Verification items for the finished model (mm, model axes). Coordinates: 2 decimals unless noted, no trailing zeros. Loops run counter-clockwise (first coordinate to the right, second up) from the corner with the lowest first, then second, coordinate; pieces in that order, holes last. Notation, with made-up numbers: (-5.5, 52.25) -> (48.5, 52.25) arc R32 cw to (48.5, 90.25) -> close; hole circle Ø3 at (-10.5, 43.5). An arc over 180 degrees is marked (long way). Answer as a JSON object with one key per item and string values. Group by question number.
Q1. Cross-section at A-A on z = 32.5. Record the boundary of the cut face in (x, y), and give its area (3 significant figures).
Q2. Cross-section at C-C on y = 1.8. Give the number of separate pieces and of enclosed holes in the cut face, and give its area (3 significant figures).
Q3. Scan lines: L1, parallel to X at y = 1.2, z = -29; L2, parallel to X at y = 0.6, z = 9; L3, parallel to X at y = 0.7, z = -32.5. Record each from-to range of solid material in increasing order.
Q4. Gauge pin test, flat ends, axial feed: pin 1 Ø6.5 at (x, z) = (-42.5, 32.5) entering from +Y; pin 2 Ø0.8 at (y, z) = (1, 3) entering from -X; pin 3 Ø1 at (y, z) = (1.5, -0.5) entering from +X; pin 4 Ø0.8 at (x, y) = (2, 1) entering from +Z. Record the tip position at first contact, or that the pin passes through.
Q5. Cross-section at B-B on x = 42.5. Record the boundary of the cut face in (y, z).
```python
from build123d import *

# Parameters (mm, degrees)
EXTRUDE_1_DEPTH     = 2.5
SKETCH_3_R          = 2
CUT_EXTRUDE_1_DEPTH = 61.570207198
CUT_EXTRUDE_2_DEPTH = 61.570207198
FILLET_1_R          = 2
FILLET_2_R          = 2


with BuildPart() as part:
    # 草图2 → 凸台-拉伸1 (new body)
    with BuildSketch(Plane(origin=(0, 0, 0), x_dir=(1, 0, 0), z_dir=(0, 1, 0))):
        Polygon((-47.5, 37.5), (-30.5, 37.5), (-20, 27), (20, 27), (30.5, 37.5), (47.5, 37.5), (47.5, 26.521871089), (36.45, 22.5), (36.45, -22.5), (47.5, -26.521871089), (47.5, -37.5), (30.5, -37.5), (20, -27), (-20, -27), (-30.5, -37.5), (-47.5, -37.5), (-47.5, -26.521871089), (-36.45, -22.5), (-36.45, 22.5), (-47.5, 26.521871089), align=None)
    extrude(amount=EXTRUDE_1_DEPTH)

    # 草图3 → 切除-拉伸1 (cut, through all)
    with BuildSketch(Plane(origin=(0, 2.5, 0), x_dir=(1, 0, 0), z_dir=(0, 1, 0))):
        with Locations(Location((-42.5, -32.5, 0), (0, 0, 270))):
            Circle(SKETCH_3_R)
        with Locations(Location((42.5, -32.5, 0), (0, 0, 270))):
            Circle(SKETCH_3_R)
        with Locations(Location((42.5, 32.5, 0), (0, 0, 90))):
            Circle(SKETCH_3_R)
        with Locations(Location((-42.5, 32.5, 0), (0, 0, 90))):
            Circle(SKETCH_3_R)
    extrude(amount=-CUT_EXTRUDE_1_DEPTH, mode=Mode.SUBTRACT)

    # 草图4 → 切除-拉伸2 (cut, through all)
    with BuildSketch(Plane(origin=(0, 2.5, 0), x_dir=(1, 0, 0), z_dir=(0, 1, 0))):
        with BuildLine():
            Line((14.432710429, 17.261137554), (0, 2.828427125))
            Line((0, 2.828427125), (-14.432710429, 17.261137554))
            ThreePointArc((-14.432710429, 17.261137554), (0, 22.5), (14.432710429, 17.261137554))
        make_face()
        with BuildLine():
            Line((17.261137554, 14.432710429), (2.828427125, 0))
            Line((2.828427125, 0), (17.261137554, -14.432710429))
            ThreePointArc((17.261137554, -14.432710429), (22.5, 0), (17.261137554, 14.432710429))
        make_face()
        with BuildLine():
            Line((14.432710429, -17.261137554), (0, -2.828427125))
            Line((0, -2.828427125), (-14.432710429, -17.261137554))
            ThreePointArc((-14.432710429, -17.261137554), (0, -22.5), (14.432710429, -17.261137554))
        make_face()
        with BuildLine():
            Line((-17.261137554, 14.432710429), (-2.828427125, 0))
            Line((-2.828427125, 0), (-17.261137554, -14.432710429))
            ThreePointArc((-17.261137554, -14.432710429), (-22.5, 0), (-17.261137554, 14.432710429))
        make_face()
        Polygon((-17.261137554, 25.402553145), (-34.014066988, 5.737935313), (-26.260100349, 5.737935313), align=None)
        Polygon((-32.876818547, 14.112219282), (-26.260100349, 27), (-32.876818547, 33.858987655), align=None)
        Polygon((26.260100349, 27), (32.876818547, 33.858987655), (32.876818547, 14.112219282), align=None)
        Polygon((34.014066988, 5.737935313), (26.260100349, 5.737935313), (17.261137554, 25.402553145), align=None)
        Polygon((32.876818547, -14.112219282), (26.260100349, -27), (32.876818547, -33.858987655), align=None)
        Polygon((17.261137554, -25.402553145), (34.014066988, -5.737935313), (26.260100349, -5.737935313), align=None)
        Polygon((-26.260100349, -27), (-32.876818547, -33.858987655), (-32.876818547, -14.112219282), align=None)
        Polygon((-34.014066988, -5.737935313), (-26.260100349, -5.737935313), (-17.261137554, -25.402553145), align=None)
    extrude(amount=-CUT_EXTRUDE_2_DEPTH, mode=Mode.SUBTRACT)

    # 圆角1
    fillet_1_edges = [part.edges().sort_by_distance(p)[0] for p in [
        (-32.876818547, 1.25, -14.112219282),
        (-32.876818547, 1.25, -33.858987655),
        (-26.260100349, 1.25, -27),
        (32.876818547, 1.25, -14.112219282),
        (26.260100349, 1.25, -27),
        (32.876818547, 1.25, -33.858987655),
        (17.261137554, 1.25, -25.402553145),
        (34.014066988, 1.25, -5.737935313),
        (26.260100349, 1.25, -5.737935313),
        (32.876818547, 1.25, 14.112219282),
        (32.876818547, 1.25, 33.858987655),
        (26.260100349, 1.25, 27),
        (14.432710429, 1.25, 17.261137554),
        (-14.432710429, 1.25, 17.261137554),
        (0, 1.25, 2.828427125),
        (17.261137554, 1.25, -14.432710429),
        (17.261137554, 1.25, 14.432710429),
        (2.828427125, 1.25, 0),
        (-17.261137554, 1.25, -25.402553145),
        (-26.260100349, 1.25, -5.737935313),
        (-34.014066988, 1.25, -5.737935313),
        (-17.261137554, 1.25, 14.432710429),
        (-17.261137554, 1.25, -14.432710429),
        (-2.828427125, 1.25, 0),
        (-17.261137554, 1.25, 25.402553145),
        (-34.014066988, 1.25, 5.737935313),
        (-26.260100349, 1.25, 5.737935313),
        (-32.876818547, 1.25, 14.112219282),
        (-26.260100349, 1.25, 27),
        (-32.876818547, 1.25, 33.858987655),
        (17.261137554, 1.25, 25.402553145),
        (26.260100349, 1.25, 5.737935313),
        (34.014066988, 1.25, 5.737935313),
        (-14.432710429, 1.25, -17.261137554),
        (14.432710429, 1.25, -17.261137554),
        (0, 1.25, -2.828427125),
    ]]
    fillet(fillet_1_edges, radius=FILLET_1_R)

    # 圆角2
    fillet_2_edges = [part.edges().sort_by_distance(p)[0] for p in [
        (30.5, 1.25, 37.5),
        (20, 1.25, 27),
        (-20, 1.25, 27),
        (-30.5, 1.25, 37.5),
        (-47.5, 1.25, 37.5),
        (-47.5, 1.25, 26.521871089),
        (-36.45, 1.25, 22.5),
        (-36.45, 1.25, -22.5),
        (-47.5, 1.25, -26.521871089),
        (-47.5, 1.25, -37.5),
        (-30.5, 1.25, -37.5),
        (-20, 1.25, -27),
        (20, 1.25, -27),
        (30.5, 1.25, -37.5),
        (47.5, 1.25, -37.5),
        (47.5, 1.25, -26.521871089),
        (36.45, 1.25, -22.5),
        (36.45, 1.25, 22.5),
        (47.5, 1.25, 26.521871089),
        (47.5, 1.25, 37.5),
    ]]
    fillet(fillet_2_edges, radius=FILLET_2_R)


solid = part.part
```
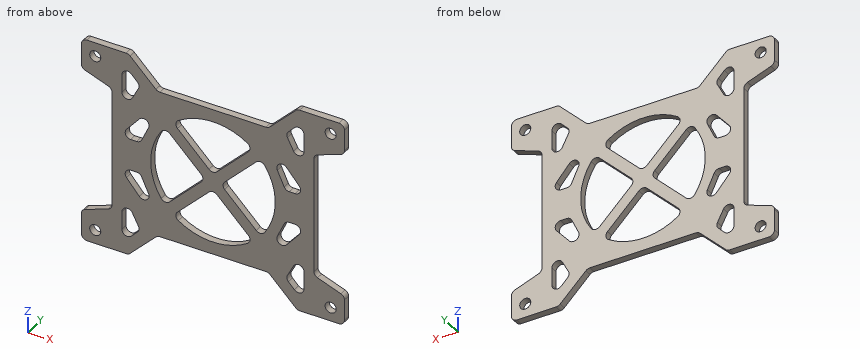
Computed values:
{
 "1": {"outline": "(-47.5, 0) -> (-44.5, 0) -> (-44.5, 2.5) -> (-47.5, 2.5) -> close; (-40.5, 0) -> (-25.5, 0) -> (-25.5, 2.5) -> (-40.5, 2.5) -> close; (25.5, 0) -> (40.5, 0) -> (40.5, 2.5) -> (25.5, 2.5) -> close; (44.5, 0) -> (47.5, 0) -> (47.5, 2.5) -> (44.5, 2.5) -> close", "area": "90.0 mm²"},
 "2": {"separate pieces": "1", "enclosed holes": "16", "area": "3,300 mm²"},
 "3": {"L1": "x = -47.5 to -32.87, -28.19 to -22, 22 to 28.19, 32.87 to 47.5", "L2": "x = -36.45 to -31.23, -24.77 to -20.62, -11.83 to -6.17, 6.17 to 11.83, 20.62 to 24.77, 31.23 to 36.45", "L3": "x = -47.5 to -44.5, -40.5 to -25.5, 25.5 to 40.5, 44.5 to 47.5"},
 "4": {"pin 1": "stops at y = 2.5", "pin 2": "stops at x = -36.45", "pin 3": "stops at x = 36.45", "pin 4": "stops at z = 27"},
 "5": {"outline": "(0, -37.5) -> (2.5, -37.5) -> (2.5, -34.5) -> (0, -34.5) -> close; (0, -30.5) -> (2.5, -30.5) -> (2.5, -24.7) -> (0, -24.7) -> close; (0, 24.7) -> (2.5, 24.7) -> (2.5, 30.5) -> (0, 30.5) -> close; (0, 34.5) -> (2.5, 34.5) -> (2.5, 37.5) -> (0, 37.5) -> close"}
}
